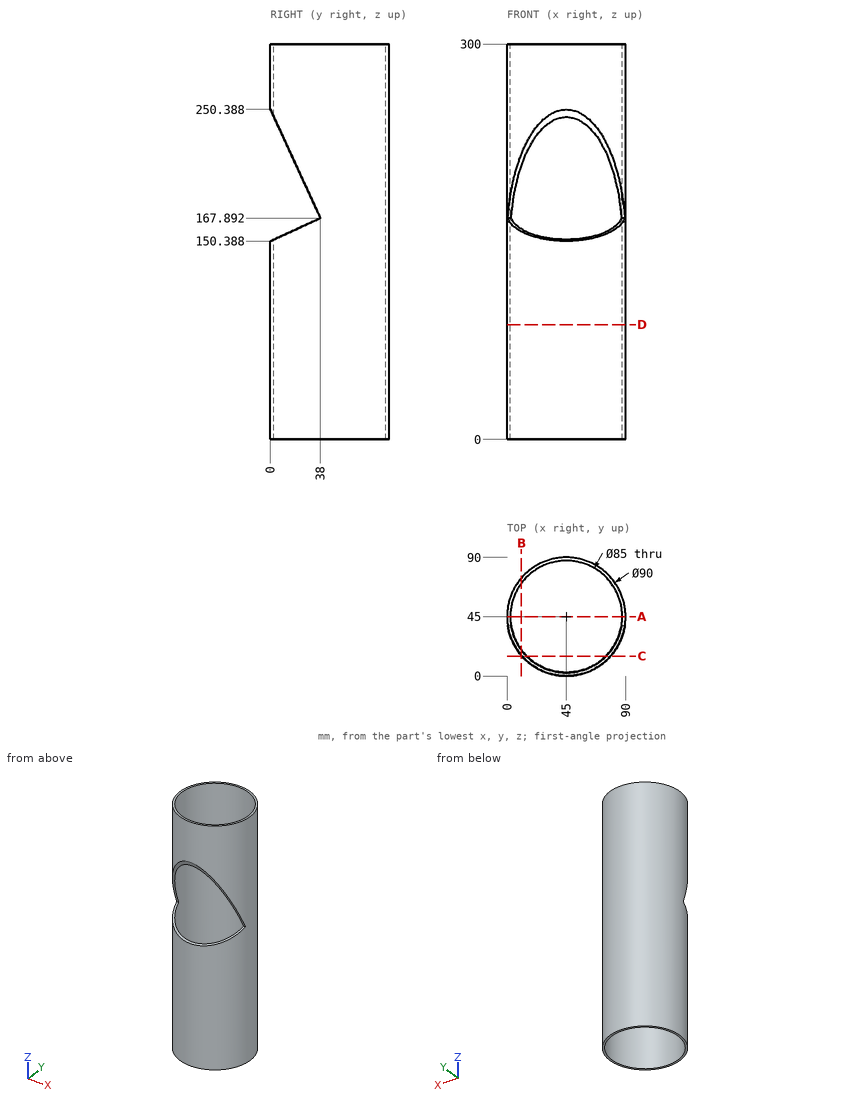
Check sheet for the drawn part. Datum: minimum x, y, z corner. Units: mm. Round coordinates to 2 decimals unless told otherwise and drop trailing zeros. Loops run counter-clockwise (first coordinate to the right, second up) from the corner with the lowest first, then second, coordinate; pieces in that order, holes last. Notation, with made-up numbers: M 25,48 L 35,48 A33 ccw 35,86 Z; hole C 22,37.5 d9. An arc over 180 degrees is marked long. One line per question, with ' | ' between items. Start each with the question number.
Item 1: Section check C-C (y = 15). Record the boundary of the cut face in (x, z) (1 decimal).
Item 2: Scan lines: probe 1 along Y at (x, z) = (45, 91.5); probe 2 along Y at (x, z) = (70, 72.5) (1 decimal); probe 3 along Y at (x, z) = (45, 239.5). Record each from-to range of solid material in increasing order.
Item 3: Section check D-D (z = 87). Record the boundary of the cut face in (x, y).
Item 4: Gauge pin test, flat ends, axial feed: pin 1 Ø5 at (x, z) = (48, 144.5) entering from -Y; pin 2 Ø6 at (y, z) = (57.5, 38.5) entering from +X (1 decimal); pin 3 Ø10 at (x, y) = (13, 33) entering from -Z; pin 4 Ø1 at (y, z) = (44.5, 181) entering from -X. Record the tip position at first contact, or that the pin passes through.
Item 5: Section check A-A (y = 45). Record the boundary of the cut face in (x, z).
Item 6: Section check B-B (x = 11). Record the boundary of the cut face in (y, z) (1 decimal), and give its area (3 significant figures).
Worked out:
1) outline: M 11.5,0 L 14.9,0 L 14.9,157.3 L 11.5,157.3 Z; M 11.5,217.8 L 14.9,217.8 L 14.9,300 L 11.5,300 Z; M 75.1,0 L 78.5,0 L 78.5,157.3 L 75.1,157.3 Z; M 75.1,217.8 L 78.5,217.8 L 78.5,300 L 75.1,300 Z
2) probe 1: 0 to 2.5, 87.5 to 90 | probe 2: 7.6 to 10.6, 79.4 to 82.4 | probe 3: 87.5 to 90
3) outline: C 45,45 d90; hole C 45,45 d85
4) pin 1: y = 0 | pin 2: x = 89 | pin 3: through | pin 4: x = 0
5) outline: M 0,0 L 2.5,0 L 2.5,300 L 0,300 Z; M 87.5,0 L 90,0 L 90,300 L 87.5,300 Z
6) outline: M 15.5,0 L 19.5,0 L 19.5,159.4 L 15.5,157.5 Z; M 15.5,216.7 L 19.5,208.1 L 19.5,300 L 15.5,300 Z; M 70.5,0 L 74.5,0 L 74.5,300 L 70.5,300 Z | area: 2,170 mm^2
